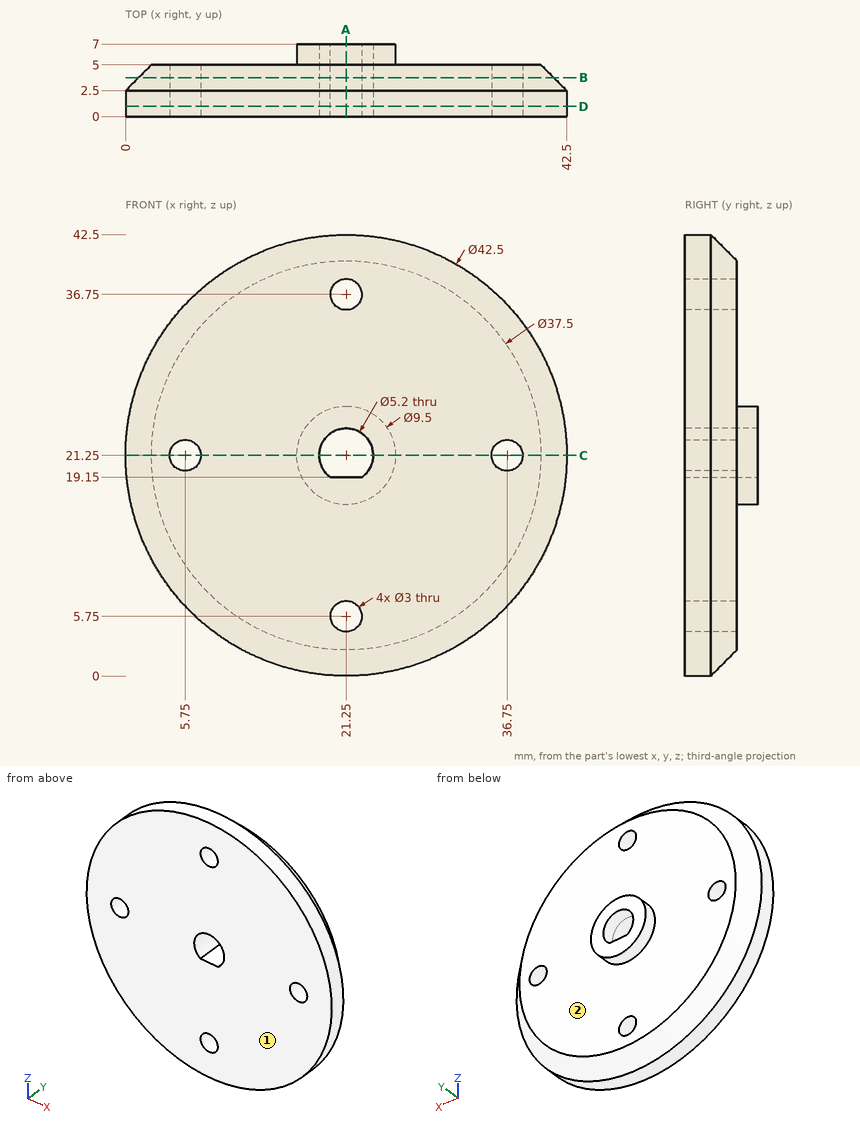
Can you work these out from the drawing? Everything is in mm from the part's minimum corner. A direction names the side the tool comes from. Round coordinates to 2 decimals unless told otherwise and drop trailing zeros. Write each loop counter-clockwise with the first axis right and the second up, starting at its lowest first coordinate (ties: lowest second). Pieces come first, ordered by that corner, then holes.
1. Suppose I cut it at C-C (z = 21.25). List the corners of the cut face in (x, y) for me, and give its area (3 significant figures).
2. For the marked faces 1 and 2, which set-ups out of +Z, -Z, +X, -X, +Y, -Y let a thin tool reach every point of the face, with its end or its side?
3. Suppose I cut it at A-A (x = 21.25). List the corners of the cut face in (y, z) for me, and give its area (3 significant figures).
4. Suppose I cut it at B-B (y = 3.75). List the corners of the cut face in (x, z) for me.
5. I need wall thicknesses on L1, parallel to X at y = 2.45, z = 21.25; L2, parallel to X at y = 5.85, z = 21.25; L3, parallel to Y at x = 24, z = 27.5. Which ranges of each line are inside material? Lowest first, please.
6. Will these pins go through, and if not, where does the flat tip stop? pin 1 Ø4 at (x, z) = (21.25, 21.25) entering from -Y; pin 2 Ø3 at (x, y) = (5, 5.5) entering from -Z; pin 3 Ø4 at (y, z) = (6, 5) entering from -X; pin 4 Ø3.5 at (x, z) = (21.25, 36.75) entering from +Y.
7. Suppose I cut it at D-D (y = 1). List the corners of the cut face in (x, z) for me, and give its area (3 significant figures).
Answer sheet:
1. outline: (0, 0) - (4.25, 0) - (4.25, 5) - (2.5, 5) - (0, 2.5) - close; (7.25, 0) - (18.65, 0) - (18.65, 7) - (16.5, 7) - (16.5, 5) - (7.25, 5) - close; (23.85, 0) - (35.25, 0) - (35.25, 5) - (26, 5) - (26, 7) - (23.85, 7) - close; (38.25, 0) - (42.5, 0) - (42.5, 2.5) - (40, 5) - (38.25, 5) - close
1. area: 159 mm2
2. face 1: +Z, -Z, +X, -X, -Y
2. face 2: +Y
3. outline: (0, 0) - (2.5, 0) - (5, 2.5) - (5, 4.25) - (0, 4.25) - close; (0, 7.25) - (5, 7.25) - (5, 16.5) - (7, 16.5) - (7, 19.15) - (0, 19.15) - close; (0, 23.85) - (7, 23.85) - (7, 26) - (5, 26) - (5, 35.25) - (0, 35.25) - close; (0, 38.25) - (5, 38.25) - (5, 40) - (2.5, 42.5) - (0, 42.5) - close
3. area: 162 mm2
4. outline: circle Ø40 at (21.25, 21.25); hole circle Ø3 at (5.75, 21.25); hole (19.72, 19.15) - (22.78, 19.15) arc R2.6 ccw (long way) to start; hole circle Ø3 at (21.25, 5.75); hole circle Ø3 at (21.25, 36.75); hole circle Ø3 at (36.75, 21.25)
5. L1: x = 0 to 4.25, 7.25 to 18.65, 23.85 to 35.25, 38.25 to 42.5
5. L2: x = 16.5 to 18.65, 23.85 to 26
5. L3: y = 0 to 5
6. pin 1: passes through
6. pin 2: stops at z = 9.3
6. pin 3: stops at x = 9.09
6. pin 4: stops at y = 5
7. outline: circle Ø42.5 at (21.25, 21.25); hole circle Ø3 at (5.75, 21.25); hole (19.72, 19.15) - (22.78, 19.15) arc R2.6 ccw (long way) to start; hole circle Ø3 at (21.25, 5.75); hole circle Ø3 at (21.25, 36.75); hole circle Ø3 at (36.75, 21.25)
7. area: 1,370 mm2
